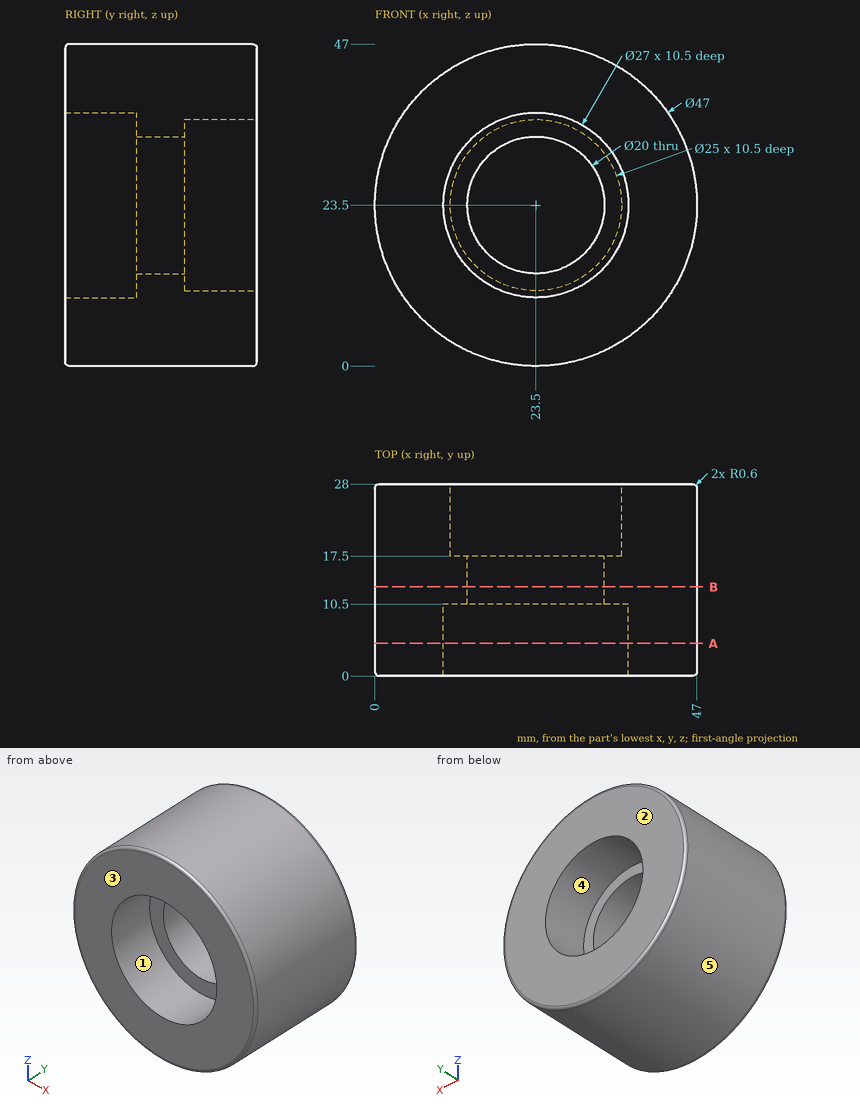
Drawing for the job (mm, zero at the part's lowest x, y, z). A direction names the side the tool comes from. Round coordinates to 2 decimals unless told otherwise and drop trailing zeros. Write each loop counter-clockwise with the first axis right and the second up, starting at its lowest first coordinate (ties: lowest second). Pieces come first, ordered by that corner, then holes. Notation, with made-up numbers: M 12,39 L 37,39 A17 ccw 37,53 Z; hole C 16,-18 d11. An arc over 180 degrees is marked long. Answer as a JSON object with one key per item and string values. Group by question number.
(1) Cut at B-B (y = 13). Give the cut face in (x, z).
(2) Flat gauge pins, fed straight in: pin 1 (23 mm diameter, centred on x = 23.5, z = 23.5, fed in from -Y); pin 2 (10 mm diameter, centred on y = 11.5, z = 6.5, fed in from -X); pin 3 (5 mm diameter, centred on x = 41.5, y = 20.5, fed in from -Z); pin 4 (5 mm diameter, centred on x = 7, z = 41.5, fed in from +Y). Where does each tip first touch, or does it go through?
(3) Which spindle directions (+Z, -Z, +X, -X, +Y, -Y) get a long thin tool onto all of the face, cutting with end or side? Do the marked faces 1 and 2. Say none if no direction does.
(4) Cut at A-A (y = 4.75). Give the cut face in (x, z), and give its area (3 significant figures).
(5) Mould opens along Z. For the marked faces 3, 4 and 5 say: pulls with the +Z half, pulls with the -Z half, needs draft (parallel to the pull), parting line crosses it, or undercut.
(6) Drill centre lines: L1, parallel to Z at x = 23.5, y = 21; L2, parallel to X at y = 15, z = 23; L3, parallel to Z at x = 23.5, y = 12.25. Where is each one in solid material? Low to high.
Responses:
{
 "1": {"outline": "C 23.5,23.5 d47; hole C 23.5,23.5 d20"},
 "2": {"pin 1": "stops at y = 10.5", "pin 2": "stops at x = 3.29", "pin 3": "stops at z = 5.84", "pin 4": "stops at y = 28"},
 "3": {"face 1": "-Y", "face 2": "+Z, -Z, +X, -X, +Y"},
 "4": {"outline": "C 23.5,23.5 d47; hole C 23.5,23.5 d27", "area": "1,160 mm2"},
 "5": {"face 3": "needs draft", "face 4": "undercut", "face 5": "parting line crosses it"},
 "6": {"L1": "z = 0 to 11, 36 to 47", "L2": "x = 0.01 to 13.51, 33.49 to 46.99", "L3": "z = 0 to 13.5, 33.5 to 47"}
}
